Build history of the part. All positions in model axes, mm. Face numbers are marked on the shaded views. A direction names the side the tool comes from. Coordinates: 2 decimals unless noted, no trailing zeros. Write each loop counter-clockwise with the first axis right and the second up, starting at its lowest first coordinate (ties: lowest second). Pieces come first, ordered by that corner, then holes. Notation, with made-up numbers: M -12,58 L 18,58 A15 ccw 18,63 Z; hole C 13.5,7 d6. An arc over 180 degrees is marked long. Use CSV: the item, a comma, the result in double quotes. Start each with the question number.
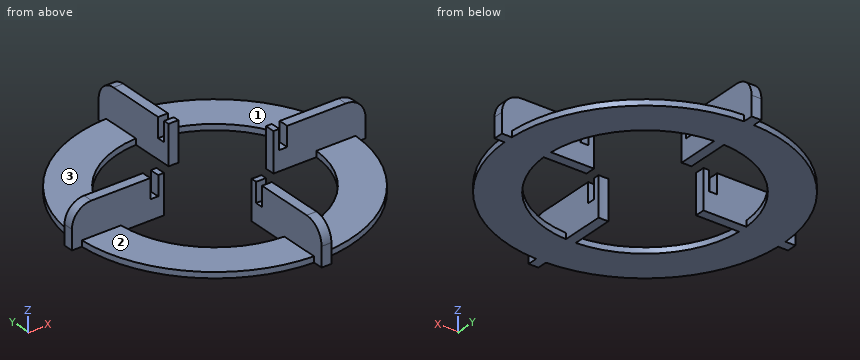
```python
from build123d import *

# Parameters (mm, degrees)
SKETCH1_W           = 72.5
SKETCH1_H           = 5
SKETCH1_W_2         = 5
SKETCH1_H_2         = 72.5
BOSS_EXTRUDE1_DEPTH = 20
SKETCH2_R           = 70
SKETCH2_R_2         = 50
BOSS_EXTRUDE2_DEPTH = 3
SKETCH3_R           = 35
SKETCH3_R_2         = 31
CUT_EXTRUDE1_DEPTH  = 10
SKETCH4_R           = 28
CUT_EXTRUDE2_DEPTH  = 21
FILLET1_R           = 10
FILLET2_R           = 10
FILLET3_R           = 10
FILLET4_R           = 10


with BuildPart() as part:
    # Sketch1 → Boss-Extrude1 (new body)
    with BuildSketch(Plane.XY):
        with Locations((-38.75, 0)):
            Rectangle(SKETCH1_W, SKETCH1_H)
        with Locations((38.75, 0)):
            Rectangle(SKETCH1_W, SKETCH1_H)
        with Locations((0, 38.75)):
            Rectangle(SKETCH1_W_2, SKETCH1_H_2)
        with Locations((0, -38.75)):
            Rectangle(SKETCH1_W_2, SKETCH1_H_2)
        Rectangle(SKETCH1_W_2, SKETCH1_H)
    extrude(amount=BOSS_EXTRUDE1_DEPTH)

    # Sketch2 → Boss-Extrude2 (add)
    with BuildSketch(Plane(origin=(0, 0, 0), x_dir=(-1, 0, 0), z_dir=(0, 0, -1))):
        Circle(SKETCH2_R)
        Circle(SKETCH2_R_2, mode=Mode.SUBTRACT)
    extrude(amount=-BOSS_EXTRUDE2_DEPTH)

    # Sketch3 → Cut-Extrude1 (cut)
    with BuildSketch(Plane.XY.offset(20)):
        Circle(SKETCH3_R)
        Circle(SKETCH3_R_2, mode=Mode.SUBTRACT)
    extrude(amount=-CUT_EXTRUDE1_DEPTH, mode=Mode.SUBTRACT)

    # Sketch4 → Cut-Extrude2 (cut, through all)
    with BuildSketch(Plane.XY.offset(20)):
        Circle(SKETCH4_R)
    extrude(amount=-CUT_EXTRUDE2_DEPTH, mode=Mode.SUBTRACT)

    # Fillet1
    fillet1_edges = [part.edges().sort_by_distance(p)[0] for p in [
        (0, 75, 20),
    ]]
    fillet(fillet1_edges, radius=FILLET1_R)

    # Fillet2
    fillet2_edges = [part.edges().sort_by_distance(p)[0] for p in [
        (75, 0, 20),
    ]]
    fillet(fillet2_edges, radius=FILLET2_R)

    # Fillet3
    fillet3_edges = [part.edges().sort_by_distance(p)[0] for p in [
        (-75, 0, 20),
    ]]
    fillet(fillet3_edges, radius=FILLET3_R)

    # Fillet4
    fillet4_edges = [part.edges().sort_by_distance(p)[0] for p in [
        (0, -75, 20),
    ]]
    fillet(fillet4_edges, radius=FILLET4_R)


solid = part.part
```
1. Slice it at B-B (y = -11). List the corners of the cut face in (x, z) (3 decimals).
2. Slice it at A-A (z = 5.5). List the corners of the cut face in (x, y), and give its area (3 significant figures).
3. 3-axis set-ups, long thin cutter, end or side, ignore diameter. For the marked faces 1, 2 and 3: which of +Z, -Z, +X, -X, +Y, -Y reach the whole face in a straight line?
4. Flat gauge pins, fed straight in: pin 1 (1.2 mm diameter, centred on x = 0.5, y = -34, fed in from +Z); pin 2 (2 mm diameter, centred on y = -51.5, z = 2.5, fed in from +X); pin 3 (12 mm diameter, centred on x = -58.5, y = -35.5, fed in from -Z); pin 4 (5 mm diameter, centred on x = 46.5, z = 2, fed in from +Y). Where does each tip first touch, or does it go through?
5. Slice it at C-C (x = -44.5). List the corners of the cut face in (y, z), and give its area (3 significant figures).
6. Slice it at D-D (x = 24). List the corners of the cut face in (y, z).
7. Drill centre lines: line 1 along X through (y, z) = (-41, 19); line 2 along Z through (x, y) = (7.5, -63.5). Where is each one in solid material? Low to high. Write a range as from..to.
Established:
1,outline,"M -69.13,0 L -48.775,0 L -48.775,3 L -69.13,3 Z; M 48.775,0 L 69.13,0 L 69.13,3 L 48.775,3 Z"
2,outline,"M -75,-2.5 L -27.89,-2.5 A28 cw -27.89,2.5 L -75,2.5 Z; M -2.5,-75 L 2.5,-75 L 2.5,-27.89 A28 cw -2.5,-27.89 Z; M -2.5,27.89 A28 cw 2.5,27.89 L 2.5,75 L -2.5,75 Z; M 27.89,-2.5 L 75,-2.5 L 75,2.5 L 27.89,2.5 A28 cw Z"
2,area,"941 mm2"
3,face 1,"+Z, +X, +Y"
3,face 2,"+Z, -X, -Y"
3,face 3,"+Z, -X, +Y"
4,pin 1,"stops at z = 10"
4,pin 2,"stops at x = 48.47"
4,pin 3,"stops at z = 0"
4,pin 4,"stops at y = 54.44"
5,outline,"M -54.03,0 L -22.8,0 L -22.8,3 L -54.03,3 Z; M -2.5,0 L 2.5,0 L 2.5,20 L -2.5,20 Z; M 22.8,0 L 54.03,0 L 54.03,3 L 22.8,3 Z"
5,area,"287 mm2"
6,outline,"M -65.76,0 L -43.86,0 L -43.86,3 L -65.76,3 Z; M 43.86,0 L 65.76,0 L 65.76,3 L 43.86,3 Z"
7,line 1,"x = -2.5..2.5"
7,line 2,"z = 0..3"
